CAD build for the part. Positions are in the model's coordinates, mm. A direction names the side the tool comes from. Round coordinates to 2 decimals unless told otherwise and drop trailing zeros.
Autodesk Inventor part; units mm, degrees
ref_plane "YZ Plane" through (0, 0, 0) normal (1, 0, 0) x (0, 1, 0)
ref_plane "XZ Plane" through (0, 0, 0) normal (0, 1, 0) x (-1, 0, 0)
ref_plane "XY Plane" through (0, 0, 0) normal (0, 0, 1) x (1, 0, 0)
sketch "Sketch1" plane through (0, 0, 0) normal (0, 1, 0) x (-1, 0, 0)
  circle A0 centre (0, 0) radius 50.8
  dimension "d0" = 101.6
extrude "Extrusion1" add sketch "Sketch1" along normal blind 7.62
sketch "Sketch2" plane through (0, 7.62, 0) normal (0, 1, 0) x (1, 0, 0)
  circle A0 centre (0, 0) radius 49.2125
  circle A1 centre (0, 0) radius 50.8
  dimension "d3" = 98.425
extrude "Extrusion2" cut sketch "Sketch2" against normal blind 3.175
sketch "Sketch3" plane through (0, 7.62, 0) normal (0, 1, 0) x (1, 0, 0)
  circle A0 centre (0, 0) radius 50.9584
extrude "Extrusion3" add sketch "Sketch3" along normal blind 7.62
sketch "Sketch4" plane through (0, 15.24, 0) normal (0, 1, 0) x (1, 0, 0)
  point P0 (0, 0)
sketch "Sketch5" plane through (0, 15.24, 0) normal (0, 1, 0) x (1, 0, 0)
  circle A0 centre (0, 0) radius 49.2125
  circle A1 centre (0, 0) radius 50.9584
  dimension "d8" = 98.425
extrude "Extrusion4" cut sketch "Sketch5" against normal blind 3.175
sketch "Sketch6" plane through (0, 15.24, 0) normal (0, 1, 0) x (1, 0, 0)
  circle A0 centre (0, 0) radius 50.8
  dimension "d11" = 101.6
extrude "Extrusion5" add sketch "Sketch6" along normal blind 5.08
sketch "Sketch7" plane through (0, 0, 0) normal (0, -1, 0) x (1, 0, 0)
  circle A0 centre (0, 0) radius 57.15
  dimension "d14" = 114.3
extrude "Extrusion6" add sketch "Sketch7" along normal blind 6.096
chamfer "Chamfer1" distance 2.54 angle 45 1 edges at (-50.8, 20.32, 0)
sketch "Sketch8" plane through (0, -6.096, 0) normal (0, -1, 0) x (1, 0, 0)
  circle A0 centre (0, 0) radius 50.8
  circle A1 centre (53.975, 0) radius 1.7526
  circle A2 centre (26.9875, 46.7437) radius 1.7526
  circle A3 centre (-26.9875, 46.7437) radius 1.7526
  circle A4 centre (-53.975, 0) radius 1.7526
  circle A5 centre (-26.9875, -46.7437) radius 1.7526
  circle A6 centre (26.9875, -46.7437) radius 1.7526
  circle A7 centre (46.7437, 26.9875) radius 1.7526
  circle A8 centre (26.9875, 46.7437) radius 1.7526
  circle A9 centre (0, 53.975) radius 1.7526
  circle A10 centre (-26.9875, 46.7437) radius 1.7526
  circle A11 centre (-46.7437, 26.9875) radius 1.7526
  circle A12 centre (-53.975, 0) radius 1.7526
  circle A13 centre (-46.7437, -26.9875) radius 1.7526
  circle A14 centre (-26.9875, -46.7437) radius 1.7526
  circle A15 centre (0, -53.975) radius 1.7526
  circle A16 centre (26.9875, -46.7437) radius 1.7526
  circle A17 centre (46.7437, -26.9875) radius 1.7526
  dimension "d20" = 3.5052
  dimension "d21" = 53.975
  dimension "d24" = 360
  dimension "d44" = 360
extrude "Extrusion7" cut sketch "Sketch8" against normal blind 6.096 contours A1 | A2 | A3 | A4 | A5 | A6
sketch "Sketch9" plane through (0, -6.096, 0) normal (0, -1, 0) x (1, 0, 0)
  circle A0 centre (0, 0) radius 12.7
  circle A1 centre (0, 0) radius 1.27
  dimension "d28" = 25.4
  dimension "d29" = 2.54
extrude "Extrusion8" cut sketch "Sketch9" against normal blind 127 contours A1
sketch "Sketch10" plane through (0, -6.096, 0) normal (0, -1, 0) x (1, 0, 0)
  circle A0 centre (0, 0) radius 1.27
  circle A1 centre (0, 0) radius 38.1
  dimension "d33" = 76.2
extrude "Extrusion9" cut sketch "Sketch10" against normal blind 9.525
sketch "Sketch11" plane through (0, 3.429, 0) normal (0, -1, 0) x (1, 0, 0)
  circle A0 centre (0, 0) radius 12.7
  circle A1 centre (0, 0) radius 1.27
  dimension "d36" = 25.4
extrude "Extrusion10" add sketch "Sketch11" along normal blind 9.525
sketch "Sketch12" plane through (0, -6.096, 0) normal (0, -1, 0) x (1, 0, 0)
  circle A0 centre (0, 0) radius 31.75
  dimension "d39" = 63.5
extrude "Extrusion11" cut sketch "Sketch12" against normal blind 40.64
sketch "Sketch13" plane through (0, 3.429, 0) normal (0, -1, 0) x (1, 0, 0)
  point P0 (0, 0)
sketch "Sketch14" plane through (0, -6.096, 0) normal (0, -1, 0) x (1, 0, 0)
  point P0 (0, 0)
sketch "Sketch15" plane through (0, -6.096, 0) normal (0, -1, 0) x (1, 0, 0)
  circle A0 centre (0, 0) radius 46.99
  circle A1 centre (0, 0) radius 43.815
  dimension "d46" = 93.98
  dimension "d47" = 87.63
extrude "Extrusion12" cut sketch "Sketch15" against normal blind 3.175
sketch "Sketch16" plane through (0, -6.096, 0) normal (0, -1, 0) x (1, 0, 0)
  point P0 (0, 0)
properties part number "O ring Dome 2"
Item 1: 3-axis set-ups, long thin cutter, end or side, ignore diameter. For faces 1 (the cylindrical face through (-11.012, 16.492, -49.592)), 2 (the flat face through (-27, 7.62, -42)), 3 (the cylindrical face through (-57.095, -3.005, -2.513)), 4 (the flat face through (-39, -2.921, 21)): which of +Z, -Z, +X, -X, +Y, -Y reach the whole face in a straight line?
Answers follow:
face 1: +Y
face 2: none
face 3: +Y, -Y
face 4: -Y
Item 2: Two-plate mould, pull along X, no slides. Class faces 5 (the cylindrical face through (26.8, -3.1, -45)), 6 (the cylindrical face through (46.94, 6.05, -14.78)), 7 (the cylindrical face through (-9.498, -4.531, -42.773)), 8 (the flat face through (10, 20.32, 31)): released by +X, released by -X, zero draft, split by the parting line, or undercut.
Answers follow:
face 5: undercut
face 6: split by the parting line
face 7: undercut
face 8: zero draft
Item 3: Flat gauge pins, fed straight in: P1, Ø4.5, axis at x = 53.975, z = 0, coming from the +Y side; P2, Ø1.5, axis at x = 41.5, y = 5.5, coming from the +Z side; P3, Ø6, axis at x = 36, y = 10.5, coming from the +Z side. Where does each tip first touch, or does it go through?
Answers follow:
P1: stops at y = 0
P2: stops at z = 27.59
P3: stops at z = 38.83
Item 4: Cut at A-A, the plane y = -4.5. State how many separate pieces and enclosed holes the cut face has, plus the area to 3 significant figures.
Answers follow:
separate pieces: 2
enclosed holes: 8
area: 4,740 mm2
Item 5: Probe line 1 (Z direction, x = 0, y = -4) (3 decimals); line 2 (X direction, y = 0.5, z = 0.5); line 3 (Y direction, x = -3.5, z = -32). List the from-to ranges inside material, lowest first.
Answers follow:
line 1: z = -57.15 to -46.99, -43.815 to -38.1, 38.1 to 43.815, 46.99 to 57.15
line 2: x = -50.8 to -38.1, 38.1 to 50.8
line 3: y = 3.43 to 20.32
